Here's the drawing with two shaded views (mm, measured from the low corner). I have some questions. A direction names the side the tool comes from. Coordinates: 2 decimals unless noted, no trailing zeros. Write each loop counter-clockwise with the first axis right and the second up, starting at its lowest first coordinate (ties: lowest second). Pieces come first, ordered by that corner, then holes.
Item 1: If I drill on probe 1 along X at (y, z) = (2, 7.5); probe 2 along X at (y, z) = (3.9, 7.5); probe 3 along Z at (x, y) = (4, 3.75), over which ranges is the centre line in solid material (lowest first)?
Item 2: I want a section at B-B on y = 2. Please give me the cut outline in (x, z) (3 decimals).
Item 3: For P1, Ø3, axis at x = 10, y = 1.5, coming from the +Z side; P2, Ø2, axis at x = 17, z = 8.5, coming from the +Y side; P3, Ø4, axis at x = 31.5, y = 3, coming from the +Z side; P4, Ø1.6, axis at x = 32.07, z = 7.5, coming from the +Y side, each with a flat end and sliding along its axis, tell me the tip position at first contact or that it passes through.
Item 4: Thinking about a two-plate mould opening in Z: for the marked faces 4, 5 and 6, which applies, +Z half, -Z half, draft (parallel to the pull), parting line (faces both ways), or undercut?
Item 5: Which directions (+Z, -Z, +X, -X, +Y, -Y) give clear straight access to the entire face, cutting with the end or side of a thin tool? Please do the marked faces 1, 2 and 3.
Item 6: I want a section at A-A on z = 7.5. Please give me the cut outline in (x, y).
Item 7: I want a section at D-D on z = 10.5. Please give me the cut outline in (x, y) (1 decimal).
Item 8: I want a section at C-C on x = 32.5. Please give me the cut outline in (y, z).
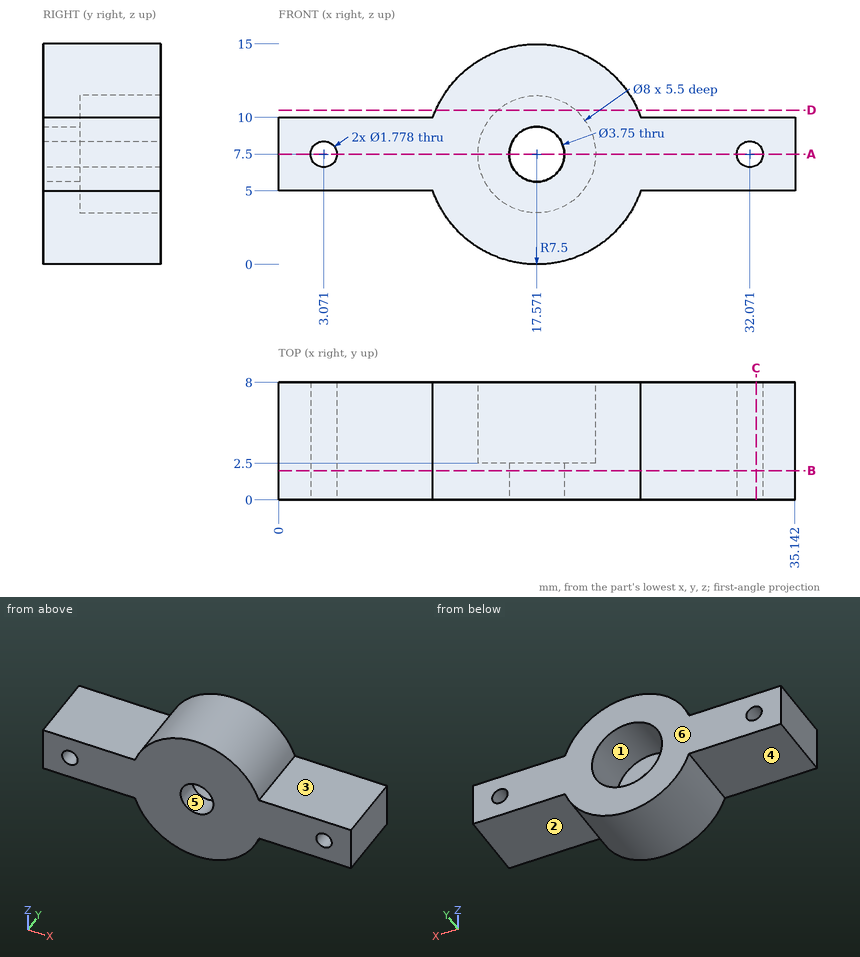
Response values:
1. probe 1: x = 0 to 2.18, 3.96 to 15.7, 19.45 to 31.18, 32.96 to 35.14
1. probe 2: x = 0 to 2.18, 3.96 to 13.57, 21.57 to 31.18, 32.96 to 35.14
1. probe 3: z = 5 to 10
2. outline: (0, 5) - (10.5, 5) arc R7.5 ccw to (24.642, 5) - (35.142, 5) - (35.142, 10) - (24.642, 10) arc R7.5 ccw to (10.5, 10) - (0, 10) - close; hole circle Ø1.778 at (3.071, 7.5); hole circle Ø3.75 at (17.571, 7.5); hole circle Ø1.778 at (32.071, 7.5)
3. P1: stops at z = 11.9
3. P2: stops at y = 2.5
3. P3: stops at z = 10
3. P4: passes through
4. face 4: -Z half
4. face 5: undercut
4. face 6: draft
5. face 1: +Y
5. face 2: -Z, +X, +Y, -Y
5. face 3: +Z, +X, +Y, -Y
6. outline: (0, 0) - (2.18, 0) - (2.18, 8) - (0, 8) - close; (3.96, 0) - (15.7, 0) - (15.7, 2.5) - (13.57, 2.5) - (13.57, 8) - (3.96, 8) - close; (19.45, 0) - (31.18, 0) - (31.18, 8) - (21.57, 8) - (21.57, 2.5) - (19.45, 2.5) - close; (32.96, 0) - (35.14, 0) - (35.14, 8) - (32.96, 8) - close
7. outline: (10.7, 0) - (24.4, 0) - (24.4, 8) - (20.2, 8) - (20.2, 2.5) - (14.9, 2.5) - (14.9, 8) - (10.7, 8) - close
8. outline: (0, 5) - (8, 5) - (8, 6.72) - (0, 6.72) - close; (0, 8.28) - (8, 8.28) - (8, 10) - (0, 10) - close
